Work out the finished part from the listing and answer in its coordinate system (mm). A direction names the side the tool comes from. Round coordinates to 2 decimals unless told otherwise and drop trailing zeros. Order: outer loops, then holes, each group sorted by start corner. A loop starts at its lowest first (then second) coordinate and runs counter-clockwise, first axis right, second up. Notation, with made-up numbers: M 83,-17.75 L 101,-17.75 A23 cw 101,1.25 Z; hole C 65.25,69 d1. An arc over 180 degrees is marked long. Answer as a JSON object with one key per item and string values. Group by question number.
from build123d import *

# Parameters (mm, degrees)
EXTRUDE_1_DEPTH      = 180
EXTRUDE_1_DEPTH_BACK = 20
SKETCH_2_W           = 42
SKETCH_2_H           = 23
CUT_EXTRUDE_1_DEPTH  = 5.5
SKETCH_4_R           = 1.5
CUT_EXTRUDE_2_DEPTH  = 5.5
SKETCH_5_W           = 2
SKETCH_5_H           = 2.2
CUT_EXTRUDE_3_DEPTH  = 225
SKETCH_6_R           = 3
CUT_EXTRUDE_4_DEPTH  = 3.5
SKETCH_7_W           = 2
SKETCH_7_H           = 1
CUT_EXTRUDE_5_DEPTH  = 200


with BuildPart() as part:
    # 草图1 → 凸台-拉伸1 (new body, two sides)
    with BuildSketch(Plane(origin=(0, 0, 0), x_dir=(0, 0, -1), z_dir=(1, 0, 0))) as extrude_1_sk:
        Polygon((-29, 0), (29, 0), (29, 9.5), (25, 9.5), (25, 4.5), (-25, 4.5), (-25, 9.5), (-29, 9.5), align=None)
    extrude(amount=EXTRUDE_1_DEPTH)
    extrude(extrude_1_sk.sketch, amount=-EXTRUDE_1_DEPTH_BACK)

    # 草图2 → 切除-拉伸1 (cut, through all)
    with BuildSketch(Plane(origin=(0, 4.5, 0), x_dir=(1, 0, 0), z_dir=(0, 1, 0))):
        with Locations((73.17, 0)):
            Rectangle(SKETCH_2_W, SKETCH_2_H)
    extrude(amount=-CUT_EXTRUDE_1_DEPTH, mode=Mode.SUBTRACT)

    # 草图4 → 切除-拉伸2 (cut, through all)
    with BuildSketch(Plane(origin=(0, 4.5, 0), x_dir=(1, 0, 0), z_dir=(0, 1, 0))):
        with Locations((66.17, 20)):
            Circle(SKETCH_4_R)
        with Locations((80.17, 20)):
            Circle(SKETCH_4_R)
        with Locations((88.17, 20)):
            Circle(SKETCH_4_R)
        with Locations((58.17, 20)):
            Circle(SKETCH_4_R)
        with Locations((88.17, -20)):
            Circle(SKETCH_4_R)
        with Locations((80.17, -20)):
            Circle(SKETCH_4_R)
        with Locations((66.17, -20)):
            Circle(SKETCH_4_R)
        with Locations((58.17, -20)):
            Circle(SKETCH_4_R)
    extrude(amount=-CUT_EXTRUDE_2_DEPTH, mode=Mode.SUBTRACT)

    # 草图5 → 切除-拉伸3 (cut)
    with BuildSketch(Plane(origin=(180, 0, 0), x_dir=(0, 0, -1), z_dir=(1, 0, 0))):
        with Locations((-26, 6.6)):
            Rectangle(SKETCH_5_W, SKETCH_5_H)
        with Locations((26, 6.6)):
            Rectangle(SKETCH_5_W, SKETCH_5_H)
    extrude(amount=-CUT_EXTRUDE_3_DEPTH, mode=Mode.SUBTRACT)

    # 草图6 → 切除-拉伸4 (cut)
    with BuildSketch(Plane(origin=(0, 0, 0), x_dir=(-1, 0, 0), z_dir=(0, -1, 0))):
        with Locations((-97.93, 5)):
            Circle(SKETCH_6_R)
        with Locations((-48.41, 5)):
            Circle(SKETCH_6_R)
        with Locations((-48.41, -5)):
            Circle(SKETCH_6_R)
        with Locations((-97.93, -5)):
            Circle(SKETCH_6_R)
    extrude(amount=-CUT_EXTRUDE_4_DEPTH, mode=Mode.SUBTRACT)

    # 草图7 → 切除-拉伸5 (cut)
    with BuildSketch(Plane(origin=(180, 0, 0), x_dir=(0, 0, -1), z_dir=(1, 0, 0))):
        with Locations((-26, 5)):
            Rectangle(SKETCH_7_W, SKETCH_7_H)
        with Locations((26, 5)):
            Rectangle(SKETCH_7_W, SKETCH_7_H)
    extrude(amount=-CUT_EXTRUDE_5_DEPTH, mode=Mode.SUBTRACT)


solid = part.part
Item 1: The mould has two halves that part along X. Classify faces 1 (the flat face through (48, 3.5, -5)), 2 (the flat face through (81, 4.5, 12)), 3 (the flat face through (-20, 3, 0)), 4 (the flat face through (180, 3, 0)): +X half, -X half, draft (parallel to the pull), parting line (faces both ways), or undercut.
Item 2: Consider L1, parallel to X at y = 1.55, z = -20; L2, parallel to X at y = 2, z = 5; L3, parallel to Z at x = 66.17, y = 2.05. Determine where each line is inside the solid, lowest interval first.
Item 3: Find section A-A (x = 48.41). Give the vertices of the cut face in (y, z).
Item 4: Find section B-B (x = 11.5). Give the vertices of the cut face in (y, z).
Item 5: Each of these flat-tipped pins is pushed along its axis until it touches: pin 1 (2 mm diameter, centred on x = 16.5, z = -1.5, fed in from +Y); pin 2 (1.8 mm diameter, centred on x = 80.17, z = 20, fed in from +Y); pin 3 (3 mm diameter, centred on x = 96.5, z = -5, fed in from -Y). Where does it stop, or does it pass through?
Item 6: A tool of negligible diameter and unlimited length cuts with its end or side. For faces 5 (the flat face through (81, 6, -27)), 6 (the flat face through (81, 5, -29)), 7 (the cylindrical face through (45.64, 1.73, -3.85)), 8 (the flat face through (73, 2, -11.5)), 9 (the flat face through (81, 5, 29)), from which of +Z, -Z, +X, -X, +Y, -Y can it reach the whole face along a straight path? Write none if from no direction.
Responses:
{
 "1": {"face 1": "undercut", "face 2": "draft", "face 3": "-X half", "face 4": "+X half"},
 "2": {"L1": "x = -20 to 56.67, 59.67 to 64.67, 67.67 to 78.67, 81.67 to 86.67, 89.67 to 180", "L2": "x = -20 to 45.41, 51.41 to 52.17, 94.17 to 94.93, 100.93 to 180", "L3": "z = -29 to -21.5, -18.5 to -11.5, 11.5 to 18.5, 21.5 to 29"},
 "3": {"outline": "M 0,-29 L 9.5,-29 L 9.5,-25 L 7.7,-25 L 7.7,-27 L 4.5,-27 L 4.5,27 L 7.7,27 L 7.7,25 L 9.5,25 L 9.5,29 L 0,29 L 0,8 L 3.5,8 L 3.5,2 L 0,2 L 0,-2 L 3.5,-2 L 3.5,-8 L 0,-8 Z"},
 "4": {"outline": "M 0,-29 L 9.5,-29 L 9.5,-25 L 7.7,-25 L 7.7,-27 L 4.5,-27 L 4.5,27 L 7.7,27 L 7.7,25 L 9.5,25 L 9.5,29 L 0,29 Z"},
 "5": {"pin 1": "stops at y = 4.5", "pin 2": "passes through", "pin 3": "stops at y = 3.5"},
 "6": {"face 5": "+X, -X", "face 6": "-Z, +X, -X, +Y, -Y", "face 7": "-Y", "face 8": "+Y, -Y", "face 9": "+Z, +X, -X, +Y, -Y"}
}
